from build123d import *

# Parameters (mm, degrees)
F0_W      = 16
F0_H      = 16
F1_DEPTH  = 0.8
F2_R      = 0.4
F3_DEPTH  = 0.6
F6_DEPTH  = 1.6
F8_R      = 8
F9_DEPTH  = 12.5
F10_R     = 1.1
F11_DEPTH = 0.801


with BuildPart() as f1:
    # F0 (on Top) → F1 (new body)
    with BuildSketch(Plane.XY):
        Rectangle(F0_W, F0_H)
    extrude(amount=F1_DEPTH)

    # F2 (on face) → F3 (join)
    with BuildSketch(Plane.XY.offset(0.8)):
        with Locations((-7.25, 7.25)):
            Circle(F2_R)
        with Locations((-7.25, 4.17)):
            Circle(F2_R)
        with Locations((-7.25, 1.09)):
            Circle(F2_R)
        with Locations((-7.25, -1.09)):
            Circle(F2_R)
        with Locations((-7.25, -4.17)):
            Circle(F2_R)
        with Locations((-7.25, -7.25)):
            Circle(F2_R)
        with Locations((-3.65, 7.25)):
            Circle(F2_R)
        with Locations((0, 7.25)):
            Circle(F2_R)
        with Locations((3.65, 7.25)):
            Circle(F2_R)
        with Locations((7.25, 7.25)):
            Circle(F2_R)
        with Locations((7.25, 4.17)):
            Circle(F2_R)
        with Locations((7.25, 1.09)):
            Circle(F2_R)
        with Locations((7.25, -1.09)):
            Circle(F2_R)
        with Locations((7.25, -4.17)):
            Circle(F2_R)
        with Locations((7.25, -7.25)):
            Circle(F2_R)
        with Locations((0, -7.25)):
            Circle(F2_R)
        with Locations((3.65, -7.25)):
            Circle(F2_R)
        with Locations((-3.65, -7.25)):
            Circle(F2_R)
    extrude(amount=F3_DEPTH)

    # F5 (on offset) → F6 (join)
    with BuildSketch(Plane.XZ.offset(5)):
        with BuildLine():
            ThreePointArc((4.5, 4.4380973526), (0, 2.8), (-4.5, 4.4380973526))
            Line((-4.5, 4.4380973526), (-6, 1.6))
            Line((-6, 1.6), (-7.25, 1.6))
            Line((-7.25, 1.6), (-7.25, 0.8))
            Line((-7.25, 0.8), (7.25, 0.8))
            Line((7.25, 0.8), (7.25, 1.6))
            Line((7.25, 1.6), (6, 1.6))
            Line((6, 1.6), (4.5, 4.4380973526))
        make_face()
    extrude(amount=F6_DEPTH)

    # F7: F1 across plane


with BuildPart() as f1_1:
    add(f1.part)
    add(f1.part.mirror(Plane.XZ))

    # F8 (on offset) → F9 (cut, symmetric)
    with BuildSketch(Plane.XZ.offset(5)):
        with Locations((0, 9.8)):
            Circle(F8_R)
    extrude(amount=F9_DEPTH, both=True, mode=Mode.SUBTRACT)

    # F10 (on face) → F11 (cut, through all)
    with BuildSketch(Plane.XY.offset(0.8)):
        with Locations((0, -3)):
            Circle(F10_R)
        with Locations((0, 1)):
            Circle(F10_R)
    extrude(amount=-F11_DEPTH, mode=Mode.SUBTRACT)


solid = f1_1.part
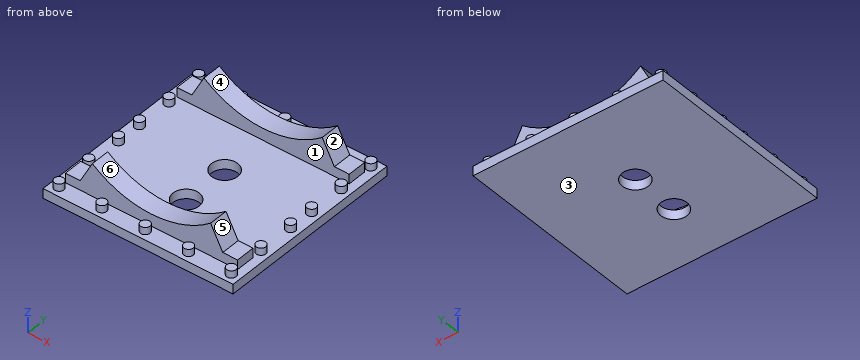
Source: CAD feature listing. Evaluate the final solid. Frame: model axes, mm. Face numbers are marked on the shaded views. A direction names the side the tool comes from. Coordinates: 2 decimals unless noted, no trailing zeros. Loops run counter-clockwise (first coordinate to the right, second up) from the corner with the lowest first, then second, coordinate; pieces in that order, holes last. Notation, with made-up numbers: M 32.25,-20 L 44.25,-20 A21 ccw 44.25,10 Z; hole C 88,16.25 d6. An arc over 180 degrees is marked long. Answer in a Markdown table with one row per item.
Q1. Section D-D on y = 1.75. Return the cut outline in (x, z), plus the area to 3 significant figures.
Answers below:
| item | result |
|---|---|
| outline | M -8,0 L -0.8,0 L -0.8,0.8 L -8,0.8 Z; M 0.8,0 L 8,0 L 8,0.8 L 0.8,0.8 Z |
| area | 11.5 mm^2 |
Q2. Draft query along X for the marked faces 3, 4, 5 and 6. Return one class per face: pulls with the +X half, pulls with the -X half, needs draft (parallel to the pull), parting line crosses it, or undercut.
Answers below:
| item | result |
|---|---|
| face 3 | needs draft |
| face 4 | undercut |
| face 5 | pulls with the +X half |
| face 6 | undercut |
Q3. First-contact query: pin 1 (0.6 mm diameter, centred on x = -7.5, y = 1, fed in from +Z); pin 2 (1.4 mm diameter, centred on x = 1.5, z = 2.5, fed in from -Y); pin 3 (0.6 mm diameter, centred on x = 6.5, y = -6, fed in from +Z). Flat tips, straight axial feed; report the tip coordinate or a pass-through.
Answers below:
| item | result |
|---|---|
| pin 1 | stops at z = 1.4 |
| pin 2 | stops at y = -6.6 |
| pin 3 | stops at z = 1.6 |
Q4. Ray query, probe 1 along Y at (x, z) = (0, 0.35); probe 2 along Y at (x, z) = (0.5, 1.35); probe 3 along Z at (x, y) = (-6.75, 5.5). Return the intervals inside material, ascending. Write a range as from..to.
Answers below:
| item | result |
|---|---|
| probe 1 | y = -8..-4.1, -1.9..-0.1, 2.1..8 |
| probe 2 | y = -6.6..-5, 5..6.6 |
| probe 3 | z = 0..1.6 |
Q5. Section A-A on z = 1.2. State how many separate pieces and enclosed holes the cut face has, plus the area to 3 significant figures.
Answers below:
| item | result |
|---|---|
| separate pieces | 20 |
| enclosed holes | 0 |
| area | 55.4 mm^2 |
Q6. Section C-C on y = 4.17. Return the cut outline in (x, z).
Answers below:
| item | result |
|---|---|
| outline | M -8,0 L 8,0 L 8,0.8 L 7.65,0.8 L 7.65,1.4 L 6.85,1.4 L 6.85,0.8 L -6.85,0.8 L -6.85,1.4 L -7.65,1.4 L -7.65,0.8 L -8,0.8 Z |
Q7. Section B-B on x = 0. Return the cut outline in (y, z).
Answers below:
| item | result |
|---|---|
| outline | M -8,0 L -4.1,0 L -4.1,0.8 L -5,0.8 L -5,1.8 L -6.6,1.8 L -6.6,0.8 L -6.85,0.8 L -6.85,1.4 L -7.65,1.4 L -7.65,0.8 L -8,0.8 Z; M -1.9,0 L -0.1,0 L -0.1,0.8 L -1.9,0.8 Z; M 2.1,0 L 8,0 L 8,0.8 L 7.65,0.8 L 7.65,1.4 L 6.85,1.4 L 6.85,0.8 L 6.6,0.8 L 6.6,1.8 L 5,1.8 L 5,0.8 L 2.1,0.8 Z |
Q8. Set-up query: the marked faces 1 and 2. Return all of +Z, -Z, +X, -X, +Y, -Y with unobstructed straight access to the full face (end or side cutting, diameter ignored); none if empty.
Answers below:
| item | result |
|---|---|
| face 1 | +Z, +X, -X |
| face 2 | +Z, +X, +Y, -Y |
